For this review, take the finished solid that the model builds, in its own axes (mm). Face numbers are marked on the shaded views. Coordinates: 2 decimals unless noted, no trailing zeros. Loops run counter-clockwise (first coordinate to the right, second up) from the corner with the lowest first, then second, coordinate; pieces in that order, holes last.
1. Take a section at A-A, the plane z = 0. State the section outline as (x, y) points, then the cut area to 3 significant figures.
2. Take a section at B-B, the plane y = 5.25. State the section outline as (x, z) points.
3. Mouldability with a two-part tool opening along Z and no side actions: class the marked faces 1, 2 and 3 as pulls with the +Z half, pulls with the -Z half, needs draft (parallel to the pull), parting line crosses it, or undercut.
4. To check wall thickness, follow probe 1 along X at (y, z) = (6.5, 0); probe 2 along Y at (x, z) = (4.75, 0.75); probe 3 along X at (y, z) = (5, -2). State the ranges of each line that lie inside material, in increasing order.
5. Clearance check with a flat-ended pin moving along its axis: P1, Ø1, axis at y = 4, z = -1.5, coming from the +X side. State where the tip first meets the part, or that it passes through.
6. Take a section at D-D, the plane x = -4.75. State the section outline as (y, z) points, then the cut area to 3 significant figures.
```python
from build123d import *

# Parameters (mm, degrees)
SKETCH_6_W             = 19.342786847
SKETCH_6_H             = 6.481709878
CUT_EXTRUDE_2_DEPTH    = 12.342618745
HOLE_WIZARD_M6_1_D     = 5
HOLE_WIZARD_M6_1_DEPTH = 28
HOLE_WIZARD_M6_1_TIP   = 1.502151548


with BuildPart() as part:
    # 草图4 → 旋转2 (revolve)
    with BuildSketch(Plane.XY, mode=Mode.PRIVATE) as revolve_2_sk:
        Polygon((0, 0), (0, 8.6), (4, 8.6), (4, 5.9), (6.85, 5.9), (6.85, 0), align=None)
    revolve(revolve_2_sk.sketch.rotate(Axis((0, 0, 0), (0, 1, 0)), 90), axis=Axis((0, 0, 0), (0, 1, 0)))

    # 草图6 → 切除-拉伸2 (cut, through all)
    with BuildSketch(Plane(origin=(0, 5.9, 0), x_dir=(1, 0, 0), z_dir=(0, 1, 0))):
        with Locations((-1.599688833, 7.240854939)):
            Rectangle(SKETCH_6_W, SKETCH_6_H)
        with Locations((-1.599688833, -7.240854939)):
            Rectangle(SKETCH_6_W, SKETCH_6_H)
    extrude(amount=-CUT_EXTRUDE_2_DEPTH, mode=Mode.SUBTRACT)

    # M6 螺纹孔1
    with Locations(Plane.ZX.offset(8.6)):
        with Locations((0, 0)):
            Hole(HOLE_WIZARD_M6_1_D / 2, depth=HOLE_WIZARD_M6_1_DEPTH)
            with Locations((0, 0, -(HOLE_WIZARD_M6_1_DEPTH + HOLE_WIZARD_M6_1_TIP / 2))):  # 118° drill point
                Cone(0, HOLE_WIZARD_M6_1_D / 2, HOLE_WIZARD_M6_1_TIP, mode=Mode.SUBTRACT)


solid = part.part
```
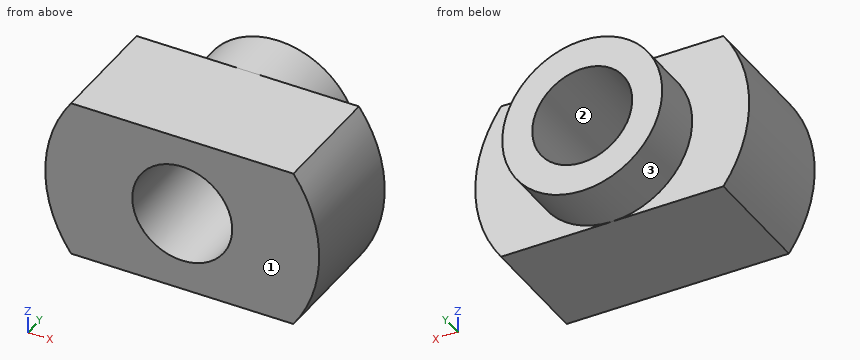
Results list:
1. outline: (-6.85, 0) - (-2.5, 0) - (-2.5, 8.6) - (-4, 8.6) - (-4, 5.9) - (-6.85, 5.9) - close; (2.5, 0) - (6.85, 0) - (6.85, 5.9) - (4, 5.9) - (4, 8.6) - (2.5, 8.6) - close
1. area: 59.4 mm2
2. outline: (-5.56, -4) - (5.56, -4) arc R6.85 ccw to (5.56, 4) - (-5.56, 4) arc R6.85 ccw to start; hole circle Ø5 at (0, 0)
3. face 1: needs draft
3. face 2: undercut
3. face 3: parting line crosses it
4. probe 1: x = -4 to -2.5, 2.5 to 4
4. probe 2: y = 0 to 5.9
4. probe 3: x = -6.55 to -1.5, 1.5 to 6.55
5. P1: stops at x = 6.78
6. outline: (0, -4) - (5.9, -4) - (5.9, 4) - (0, 4) - close
6. area: 47.2 mm2
